The model under review builds one solid part; all positions refer to its coordinate system, in mm. Face numbers are marked on the shaded views. Round coordinates to 2 decimals unless told otherwise and drop trailing zeros. Order: outer loops, then holes, each group sorted by start corner. A loop starts at its lowest first (then second) coordinate and runs counter-clockwise, first axis right, second up. Notation, with made-up numbers: (47, 14.5) -> (61, 14.5) arc R22 cw to (61, 31.5) -> close; hole circle Ø9 at (-7, 76). An arc over 180 degrees is marked (long way). Use a Markdown table: item, result. Add a question column.
Autodesk Inventor part; units mm, degrees
ref_plane "YZ Plane" through (0, 0, 0) normal (1, 0, 0) x (0, 1, 0)
ref_plane "XZ Plane" through (0, 0, 0) normal (0, 1, 0) x (-1, 0, 0)
ref_plane "XY Plane" through (0, 0, 0) normal (0, 0, 1) x (1, 0, 0)
sketch "Sketch1" plane through (0, 0, 0) normal (0, 0, 1) x (1, 0, 0)
  circle A0 centre (-12.7, 12.7) radius 38.1
  line L0 (-12.7, 12.7) -> (-12.7, 63.5)
  line L1 (-12.7, 63.5) -> (50.8, 63.5)
  line L2 (-12.7, 63.5) -> (-76.2, 63.5)
  circle A1 centre (-76.2, 63.5) radius 12.7
  circle A2 centre (50.8, 63.5) radius 12.7
  line L3 (-76.2, 76.2) -> (50.8, 76.2)
  line L4 (-86.8343, 56.5572) -> (-44.6028, -8.1284)
  line L5 (61.4343, 56.5572) -> (19.2028, -8.1284)
  point P0 (0, 0)
  dimension "d1" = 76.2
  dimension "d2" = 50.8
  dimension "d3" = 63.5
  dimension "d4" = 63.5
  dimension "d5" = 25.4
  dimension "d6" = 25.4
extrude "Extrusion2" add sketch "Sketch1" along normal blind 9.525
sketch "Sketch3" plane through (0, 0, 9.525) normal (0, 0, 1) x (1, 0, 0)
  line L0 (50.8, 76.2) -> (-76.2, 76.2) construction
  line L1 (-12.7, 76.2) -> (-12.7, -25.4) construction
  arc A0 (-44.6028, -8.1284) -> (19.2028, -8.1284) centre (-12.7, 12.7) ccw construction
  point P0 (0, 0)
  point P1 (-12.7, 0)
  dimension "d40" = 25.4
hole "Hole4" at (-12.7, 0, 9.525) direction (0, 0, -1) diameter 28.575 depth 25.4 tip angle 118
equation "\"d3\" = d4"
properties part number "bearingplaterear" material "Steel, Mild"
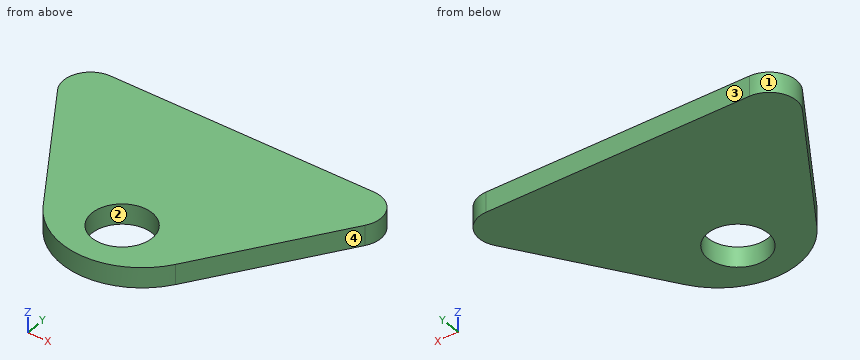
Q1. Draft analysis for pull direction X (two halves, no side actions). For the marked faces 1, 2, 3 and 4, state which applies: released by +X, released by -X, zero draft, split by the parting line, or undercut.
Q2. Add section A-A, the plane x = -12.7. Give the boundary of the cut face in (y, z) (1 decimal).
Q3. To check wall thickness, follow line 1 along Y through (x, z) = (-12.7, 7); line 2 along X through (y, z) = (-13, 1); line 3 along X through (y, z) = (0, 4.25). State the ranges of each line that lie inside material, in increasing order.
Q4. Add section D-D, the plane x = -58. Give the boundary of the cut face in (y, z) (3 decimals), then the cut area to 3 significant figures.
Q5. Add section B-B, the plane y = 0. Give the boundary of the cut face in (x, z) (1 decimal), then the cut area to 3 significant figures.
Q6. Add section C-C, the plane z = 5.25. Give the boundary of the cut face in (x, y) (1 decimal), then the cut area to 3 significant figures.
Q7. For pin 1 (3 mm diameter, centred on x = 47, z = 7.5, fed in from -Y); pin 2 (5 mm diameter, centred on x = -69.5, z = 4, fed in from -Y); pin 3 (1 mm diameter, centred on y = 42, z = 2.5, fed in from +X), all flat-tipped, find the tip position at first contact; note any pin that passes through.
Return value:
| question | item | result |
|---|---|---|
| 1 | face 1 | released by -X |
| 1 | face 2 | undercut |
| 1 | face 3 | zero draft |
| 1 | face 4 | released by +X |
| 2 | outline | (-25.4, 0) -> (-14.3, 0) -> (-14.3, 9.5) -> (-25.4, 9.5) -> close; (14.3, 0) -> (76.2, 0) -> (76.2, 9.5) -> (14.3, 9.5) -> close |
| 3 | line 1 | -25.4 to -14.29, 14.29 to 76.2 |
| 3 | line 2 | -40.83 to -18.63, -6.77 to 15.43 |
| 3 | line 3 | -49.91 to -26.99, 1.59 to 24.51 |
| 4 | outline | (12.392, 0) -> (76.2, 0) -> (76.2, 9.525) -> (12.392, 9.525) -> close |
| 4 | area | 608 mm² |
| 5 | outline | (-49.9, 0) -> (-27, 0) -> (-27, 9.5) -> (-49.9, 9.5) -> close; (1.6, 0) -> (24.5, 0) -> (24.5, 9.5) -> (1.6, 9.5) -> close |
| 5 | area | 437 mm² |
| 6 | outline | (-86.8, 56.6) -> (-44.6, -8.1) arc R38.1 ccw to (19.2, -8.1) -> (61.4, 56.6) arc R12.7 ccw to (50.8, 76.2) -> (-76.2, 76.2) arc R12.7 ccw to start; hole circle Ø28.6 at (-12.7, 0) |
| 6 | area | 9,910 mm² |
| 7 | pin 1 | y = 32.15 |
| 7 | pin 2 | y = 26.18 |
| 7 | pin 3 | x = 52.26 |
